from build123d import *

# Parameters (mm, degrees)
SKETCH1_R           = 1.75
BOSS_EXTRUDE1_DEPTH = 4
SKETCH2_W           = 130
SKETCH2_H           = 10
BOSS_EXTRUDE2_DEPTH = 0.5
CUT_EXTRUDE1_DEPTH  = 2


with BuildPart() as part:
    # Sketch1 → Boss-Extrude1 (new body)
    with BuildSketch(Plane(origin=(0, 0, 0), x_dir=(1, 0, 0), z_dir=(0, 1, 0))):
        with BuildLine():
            ThreePointArc((75, 2), (74.121320344, 4.121320344), (72, 5))
            Line((72, 5), (-72, 5))
            ThreePointArc((-72, 5), (-74.121320344, 4.121320344), (-75, 2))
            Line((-75, 2), (-75, -5))
            Line((-75, -5), (75, -5))
            Line((75, -5), (75, 2))
        make_face()
        with Locations(Location((-70, 0, 0), (0, 0, 270))):
            Circle(SKETCH1_R, mode=Mode.SUBTRACT)
        with BuildLine():
            ThreePointArc((61.75, 0), (61.237436867, -1.237436867), (60, -1.75))
            Line((60, -1.75), (-60, -1.75))
            ThreePointArc((-60, -1.75), (-61.75, 0), (-60, 1.75))
            Line((-60, 1.75), (60, 1.75))
            ThreePointArc((60, 1.75), (61.237436867, 1.237436867), (61.75, 0))
        make_face(mode=Mode.SUBTRACT)
        with Locations(Location((70, 0, 0), (0, 0, 270))):
            Circle(SKETCH1_R, mode=Mode.SUBTRACT)
    extrude(amount=BOSS_EXTRUDE1_DEPTH)

    # Sketch2 → Boss-Extrude2 (add)
    with BuildSketch(Plane(origin=(0, 4, 0), x_dir=(1, 0, 0), z_dir=(0, 1, 0))):
        Rectangle(SKETCH2_W, SKETCH2_H)
        with BuildLine():
            Line((-60, 1.75), (60, 1.75))
            ThreePointArc((60, 1.75), (61.75, 0), (60, -1.75))
            Line((60, -1.75), (-60, -1.75))
            ThreePointArc((-60, -1.75), (-61.75, 0), (-60, 1.75))
        make_face(mode=Mode.SUBTRACT)
    extrude(amount=BOSS_EXTRUDE2_DEPTH)

    # Sketch3 → Cut-Extrude1 (cut)
    with BuildSketch(Plane.XY.offset(5)):
        with BuildLine():
            Line((-58.5, 2.5), (58.5, 2.5))
            ThreePointArc((58.5, 2.5), (59.560660172, 2.939339828), (60, 4))
            Line((60, 4), (60, 4.5))
            Line((60, 4.5), (-60, 4.5))
            Line((-60, 4.5), (-60, 4))
            ThreePointArc((-60, 4), (-59.560660172, 2.939339828), (-58.5, 2.5))
        make_face()
    extrude(amount=-CUT_EXTRUDE1_DEPTH, mode=Mode.SUBTRACT)


solid = part.part
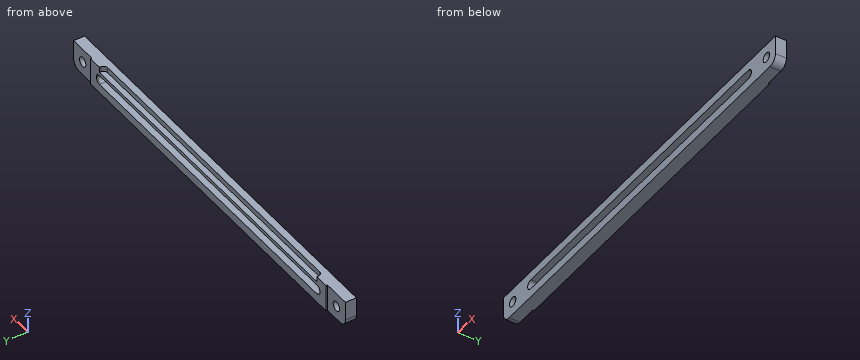
Model file for the job. Use its own axes, mm. Give positions to 0.01 mm unless a question says otherwise; leave off trailing zeros. Order: outer loops, then holes, each group sorted by start corner. A loop starts at its lowest first (then second) coordinate and runs counter-clockwise, first axis right, second up. Notation, with made-up numbers: (-26, 46.25) - (3, 46.25) arc R23 cw to (3, 82.25) - close; hole circle Ø10 at (39, -2.75). An arc over 180 degrees is marked (long way). Return JSON: item names as keys, results as strings.
1) Flat gauge pins, fed straight in: P1, Ø0.6, axis at x = 23.5, y = 3.5, coming from the +Z side; P2, Ø3, axis at x = -71.5, z = 1, coming from the +Y side; P3, Ø0.6, axis at x = 14, z = 4.5, coming from the +Y side. Where does each tip first touch, or does it go through?
Geometry says:
{"P1": "z = 3", "P2": "y = 4", "P3": "y = 2.5"}
2) Cut at B-B, the plane y = 1.35. Give the cut face in (x, z).
Geometry says:
{"outline": "(-75, -2) arc R3 ccw to (-72, -5) - (72, -5) arc R3 ccw to (75, -2) - (75, 5) - (-75, 5) - close; hole circle Ø3.5 at (-70, 0); hole (-60, -1.75) - (60, -1.75) arc R1.75 ccw to (60, 1.75) - (-60, 1.75) arc R1.75 ccw to start; hole circle Ø3.5 at (70, 0)"}
3) Cut at C-C, the plane x = -41. Give the cut face in (y, z), plus the area to 4 significant figures.
Geometry says:
{"outline": "(0, -5) - (4.5, -5) - (4.5, -1.75) - (0, -1.75) - close; (0, 1.75) - (4.5, 1.75) - (4.5, 3) - (2.5, 3) - (2.5, 5) - (0, 5) - close", "area": "25.25 mm²"}
4) Probe line 1 (X direction, y = 1.05, z = 0); line 2 (Z direction, x = -49, y = 1.7). List the from-to ranges inside material, lowest first. Write a range as from..to.
Geometry says:
{"line 1": "-75..-71.75, -68.25..-61.75, 61.75..68.25, 71.75..75", "line 2": "-5..-1.75, 1.75..5"}
5) Cut at A-A, the plane x = -70. Give the cut face in (y, z), plus the area to 3 significant figures.
Geometry says:
{"outline": "(0, -5) - (4, -5) - (4, -1.75) - (0, -1.75) - close; (0, 1.75) - (4, 1.75) - (4, 5) - (0, 5) - close", "area": "26.0 mm²"}
6) Cut at D-D, the plane z = -3.25. Give the cut face in (x, y).
Geometry says:
{"outline": "(-74.73, 0) - (74.73, 0) - (74.73, 4) - (65, 4) - (65, 4.5) - (-65, 4.5) - (-65, 4) - (-74.73, 4) - close"}
